Geometry: see drawing. Coordinates: mm, zero at the bounding-box minimum. A direction names the side the tool comes from. Coordinates: 2 decimals unless noted, no trailing zeros. Order: outer loops, then holes, each group sorted by start corner. A loop starts at its lowest first (then second) coordinate and runs counter-clockwise, first axis right, second up.
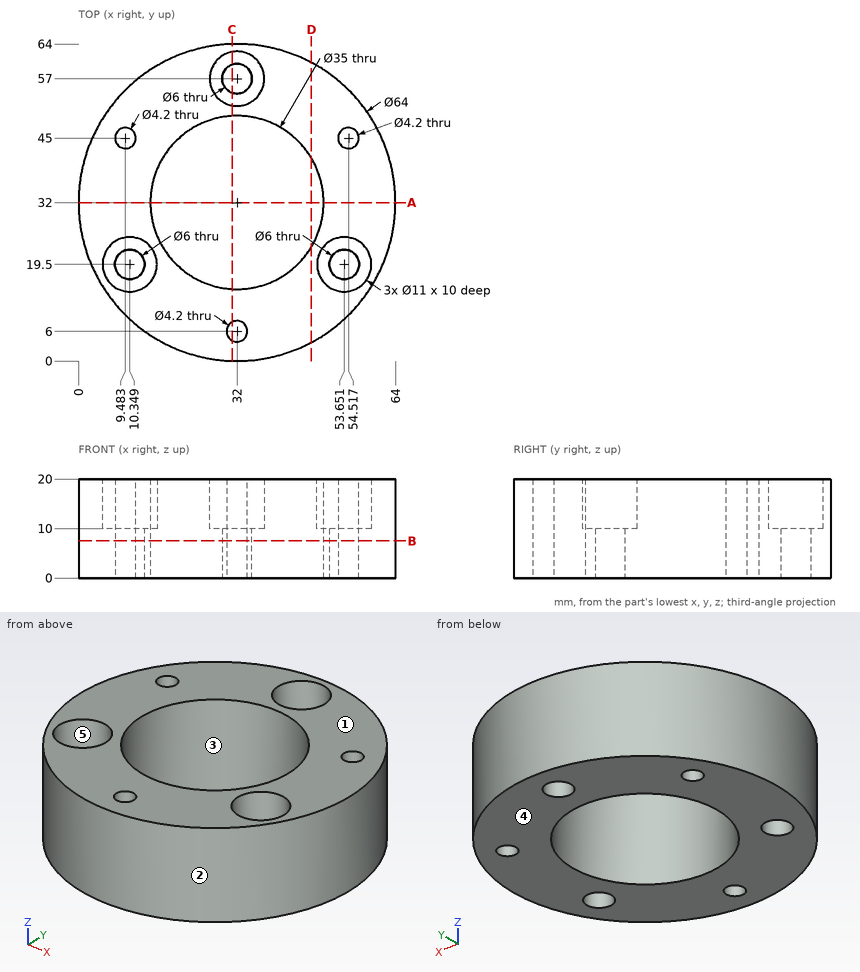
Item 1: Draft query along X for the marked faces 1, 2 and 3. Return one class per face: pulls with the +X half, pulls with the -X half, needs draft (parallel to the pull), parting line crosses it, or undercut.
Response values:
face 1: needs draft
face 2: parting line crosses it
face 3: undercut
Item 2: Cut plane A-A on y = 32. Return loops of the section in (x, z).
Response values:
outline: (0, 0) - (14.5, 0) - (14.5, 20) - (0, 20) - close; (49.5, 0) - (64, 0) - (64, 20) - (49.5, 20) - close
Item 3: Cut plane B-B on z = 7.5. Return loops of the section in (x, y).
Response values:
outline: circle Ø64 at (32, 32); hole circle Ø6 at (10.35, 19.5); hole circle Ø4.2 at (9.48, 45); hole circle Ø35 at (32, 32); hole circle Ø6 at (32, 57); hole circle Ø4.2 at (32, 6); hole circle Ø6 at (53.65, 19.5); hole circle Ø4.2 at (54.52, 45)
Item 4: Ray query, probe 1 along Y at (x, z) = (32, 9.75); probe 2 along Y at (x, z) = (32, 15.75); probe 3 along X at (y, z) = (19.5, 7.5). Return the intervals inside material, ascending.
Response values:
probe 1: y = 0 to 3.9, 8.1 to 14.5, 49.5 to 54, 60 to 64
probe 2: y = 0 to 3.9, 8.1 to 14.5, 49.5 to 51.5, 62.5 to 64
probe 3: x = 2.54 to 7.35, 13.35 to 19.75, 44.25 to 50.65, 56.65 to 61.46
Item 5: Cut plane C-C on x = 31. Return loops of the section in (y, z) (1 decimal).
Response values:
outline: (0, 0) - (4.2, 0) - (4.2, 20) - (0, 20) - close; (7.8, 0) - (14.5, 0) - (14.5, 20) - (7.8, 20) - close; (49.5, 0) - (54.2, 0) - (54.2, 10) - (51.6, 10) - (51.6, 20) - (49.5, 20) - close; (59.8, 0) - (64, 0) - (64, 20) - (62.4, 20) - (62.4, 10) - (59.8, 10) - close
Item 6: Pin query (flat end, axial travel): pin 1 Ø1.5 at (y, z) = (32.5, 6.5) entering from -X; pin 2 Ø5 at (y, z) = (18, 13.5) entering from -X; pin 3 Ø3.5 at (x, y) = (32, 55.5) entering from +Z; pin 4 Ø4 at (x, y) = (32, 6) entering from +Z (1 decimal). Return the tip coordinate at first contact, or that it passes through.
Response values:
pin 1: stops at x = 0
pin 2: stops at x = 2.14
pin 3: stops at z = 10
pin 4: passes through
Item 7: Cut plane D-D on x = 47. Return loops of the section in (y, z), then the cut area to 3 significant figures.
Response values:
outline: (3.73, 0) - (22.99, 0) - (22.99, 20) - (3.73, 20) - close; (41.01, 0) - (60.27, 0) - (60.27, 20) - (41.01, 20) - close
area: 770 mm2
Item 8: Access query for the marked faces 4 and 5. Directions: +Z, -Z, +X, -X, +Y, -Y. A direction counts if a zero-diameter tool reaches every point of the face in a straight line with its end or side. Return the directions, or none.
Response values:
face 4: -Z, +X, -X, +Y, -Y
face 5: +Z
